Autodesk Inventor part; units mm, degrees
ref_plane "YZ Plane" through (0, 0, 0) normal (1, 0, 0) x (0, 1, 0)
ref_plane "XZ Plane" through (0, 0, 0) normal (0, 1, 0) x (-1, 0, 0)
ref_plane "XY Plane" through (0, 0, 0) normal (0, 0, 1) x (1, 0, 0)
sketch "Sketch1" plane through (0, 0, 0) normal (0, 0, 1) x (1, 0, 0)
  line L0 (0, 0) -> (0, 40.5)
  line L1 (0, 40.5) -> (20, 40.5)
  line L2 (20, 40.5) -> (20, 0)
  line L3 (20, 0) -> (0, 0)
  dimension "d0" = 40.5
  dimension "d1" = 20
extrude "Extrusion1" add sketch "Sketch1" along normal blind 40
sketch "Sketch2" plane through (0, 40.5, 0) normal (0, 1, 0) x (1, 0, 0)
  line L0 (20, 0) -> (0, 0)
  line L1 (10, 0) -> (10, -10)
  circle A0 centre (10, -10) radius 5
  dimension "d4" = 10
  dimension "d5" = 10
extrude "Extrusion2" add sketch "Sketch2" along normal blind 1
sketch "Sketch3" plane through (10, 41.5, 10) normal (0, 1, 0) x (1, 0, 0)
  circle A0 centre (0, 0) radius 2
  point P0 (-10, 10)
  dimension "d8" = 4
extrude "Extrusion3" add sketch "Sketch3" along normal blind 6
fillet "Fillet1" radius 1 4 edges at (0, 20.25, 40) (20, 20.25, 40) (20, 20.25, 0) (0, 20.25, 0)
sketch "Sketch4" plane through (1, 0, 0) normal (0, -1, 0) x (1, 0, 0)
  line L0 (18, 0) -> (0, 0)
  line L1 (9, 0) -> (9, 10)
  circle A0 centre (9, 10) radius 5
  point P0 (-1, 0)
  dimension "d12" = 10
  dimension "d13" = 10
extrude "Extrusion4" add sketch "Sketch4" along normal blind 1
sketch "Sketch5" plane through (10, -1, 10) normal (0, -1, 0) x (1, 0, 0)
  circle A0 centre (0, 0) radius 2
  point P0 (-10, -10)
  dimension "d16" = 4
extrude "Extrusion5" add sketch "Sketch5" along normal blind 6
sketch "Boceto6" plane through (0, 0, 1) normal (-1, 0, 0) x (0, 0, 1)
  line L0 (-1, 0) -> (-1, 40.5)
  line L1 (-1, 40.5) -> (-1, 35.5)
  line L2 (-1, 35.5) -> (9, 35.5)
  line L3 (9, 35.5) -> (9, 29.5)
  line L4 (9, 29.5) -> (19, 29.5)
  line L5 (19, 29.5) -> (19, 35.5)
  line L6 (19, 35.5) -> (9, 35.5)
  dimension "d19" = 5
  dimension "d20" = 10
  dimension "d21" = 6
  dimension "d22" = 10
extrude "Extrusión6" cut sketch "Boceto6" against normal up to next
sketch "Boceto7" plane through (1, 0, 0) normal (0, -1, 0) x (1, 0, 0)
  line L0 (-1, 10) -> (19, 10)
  circle A0 centre (9, 10) radius 6.5
  circle A1 centre (9, 10) radius 2
  point P0 (-1, 0)
  dimension "d25" = 13
extrude "Extrusión8" add sketch "Boceto7" along normal blind 2 contours A1 L0 A0 | L0 A0 A1
sketch "Boceto8" plane through (1, 40.5, 0) normal (0, 1, 0) x (1, 0, 0)
  circle A0 centre (9, -10) radius 2
  circle A1 centre (9, -10) radius 6.5
  circle A2 centre (9, -10) radius 6.5
  circle A3 centre (9, -10) radius 2
  point P0 (-1, 0)
  dimension "d30" = 13
extrude "Extrusión9" add sketch "Boceto8" along normal blind 2
properties part number "servo_FT_SC"
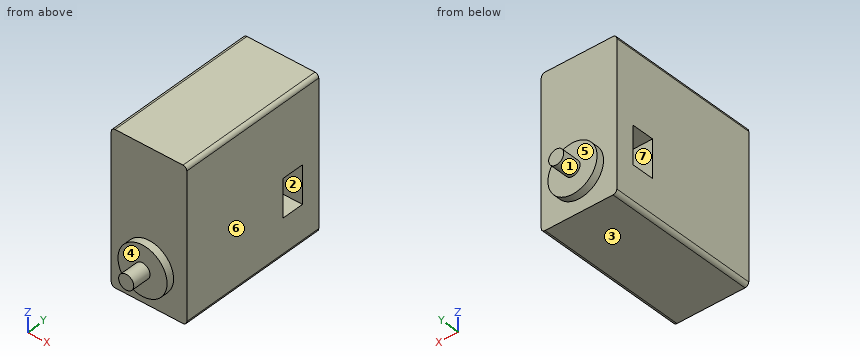
Can you work these out from the model? Positions are in its coordinate system, mm. Face numbers are marked on the shaded views. A direction names the side the tool comes from. Coordinates: 2 decimals unless noted, no trailing zeros. Order: outer loops, then holes, each group sorted by start corner. A loop starts at its lowest first (then second) coordinate and runs counter-clockwise, first axis right, second up. Notation, with made-up numbers: M -12,70 L -8,70 A25 cw -8,93 Z; hole C -17,71.5 d4. An arc over 180 degrees is marked long. Answer as CSV lines item,"result".
(1) Suppose I cut it at A-A on y = 33. Please give me the cut outline in (x, z), plus the area to 3 significant figures.
Geometry check:
outline,"M 0,1 A1 ccw 1,0 L 19,0 A1 ccw 20,1 L 20,10 L 0,10 Z; M 0,20 L 20,20 L 20,39 A1 ccw 19,40 L 1,40 A1 ccw 0,39 Z"
area,"599 mm^2"
(2) Suppose I cut it at C-C on z = 11. Please give me the cut outline in (x, y), plus the area to 3 significant figures.
Geometry check:
outline,"M 0,0 L 3.58,0 L 3.58,-2 L 8.27,-2 L 8.27,-7 L 11.73,-7 L 11.73,-2 L 16.42,-2 L 16.42,0 L 20,0 L 20,29.5 L 0,29.5 Z; M 0,35.5 L 20,35.5 L 20,40.5 L 16.42,40.5 L 16.42,42.5 L 11.73,42.5 L 11.73,47.5 L 8.27,47.5 L 8.27,42.5 L 3.58,42.5 L 3.58,40.5 L 0,40.5 Z"
area,"776 mm^2"
(3) Suppose I cut it at B-B on x = 10. Please give me the cut outline in (y, z).
Geometry check:
outline,"M -7,8 L -2,8 L -2,3.5 L 0,3.5 L 0,0 L 40.5,0 L 40.5,3.5 L 42.5,3.5 L 42.5,8 L 47.5,8 L 47.5,12 L 42.5,12 L 42.5,16.5 L 40.5,16.5 L 40.5,40 L 0,40 L 0,16.5 L -2,16.5 L -2,12 L -7,12 Z; hole M 29.5,10 L 35.5,10 L 35.5,20 L 29.5,20 Z"
(4) On a 3-axis mill with a long thin cutter (end or side, diameter ignored), from which of +Z, -Z, +X, -X, +Y, -Y can I reach the whole of each face in a straight line? I mean the marked faces 4, 5, 6 and 7. Say none if no direction works.
Geometry check:
face 4,"-Y"
face 5,"+Y"
face 6,"+Z, -Z, +X, +Y, -Y"
face 7,"+X, -X"
(5) I'm going to push flat-ended pins straight in: pin 1 (1.8 mm diameter, centred on x = 13, y = 34, fed in from -Z); pin 2 (1.5 mm diameter, centred on x = 13, z = 31.5, fed in from +Y); pin 3 (6 mm diameter, centred on x = 9.5, z = 22, fed in from -Y); pin 4 (3 mm diameter, centred on x = 3.5, z = 11, fed in from +Y). Where does each tip first touch, or does it pass through?
Geometry check:
pin 1,"z = 0"
pin 2,"y = 40.5"
pin 3,"y = 0"
pin 4,"y = 42.5"
(6) If we mould it in two halves opening along Z, with no side actions, what happens to the marked faces 1, 2 and 3? For each: released by +Z, released by -Z, zero draft, split by the parting line, or undercut.
Geometry check:
face 1,"split by the parting line"
face 2,"undercut"
face 3,"released by -Z"
(7) Please list where these lines run through material, in increasing order: L1, parallel to Z at x = 15.5, y = 33.5; L2, parallel to Y at x = 15.25, z = 13; L3, parallel to Y at x = 15, z = 17.5.
Geometry check:
L1,"0 to 10, 20 to 40"
L2,"-2 to 29.5, 35.5 to 42.5"
L3,"0 to 29.5, 35.5 to 40.5"
(8) Suppose I cut it at D-D on x = 14.25. Please give me the cut outline in (y, z).
Geometry check:
outline,"M -2,5.08 L 0,5.08 L 0,0 L 40.5,0 L 40.5,5.08 L 42.5,5.08 L 42.5,14.92 L 40.5,14.92 L 40.5,40 L 0,40 L 0,14.92 L -2,14.92 Z; hole M 29.5,10 L 35.5,10 L 35.5,20 L 29.5,20 Z"
